Geometry check sheet. Reference: the model listing, model coordinates, mm. Face numbers are marked on the shaded views. A direction names the side the tool comes from. Coordinates: 2 decimals unless noted, no trailing zeros. Write each loop counter-clockwise with the first axis right and the second up, starting at its lowest first coordinate (ties: lowest second). Pieces come first, ordered by that corner, then holes. Notation, with made-up numbers: M 6,64.5 L 31,64.5 A24 cw 31,93.5 Z; hole C 30.5,0.25 d11. An arc over 180 degrees is marked long. Answer as a JSON object with one key per item and string values. Group by question number.
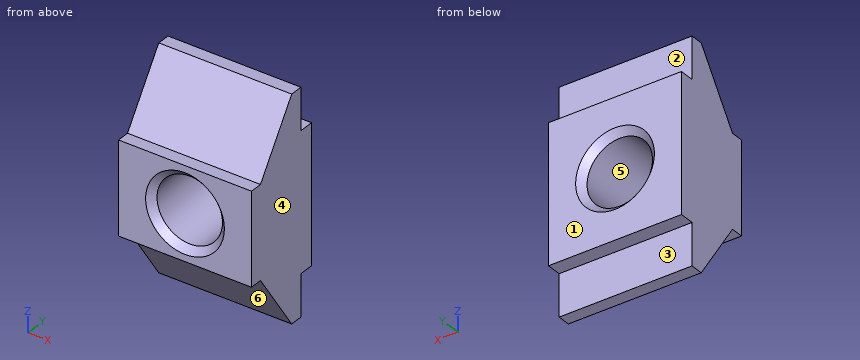
Autodesk Inventor part; units mm, degrees
ref_plane "TIN_4_XY" through (0, 8.5, 0) normal (0, 1, 0) x (1, 0, 0)
ref_plane "TIN_4_YZ" through (0, 8.5, 0) normal (1, 0, 0) x (0, 0, -1)
ref_plane "TIN_4_ZX" through (0, 8.5, 0) normal (0, 0, -1) x (0, 1, 0)
sketch "Skizze_1" plane through (0, 0, 0) normal (1, 0, 0) x (0, 1, 0)
  line L0 (5.7, 11.25) -> (1.275, 4.7)
  line L1 (1.275, 4.7) -> (0, 4.7)
  line L2 (0, 4.7) -> (0, -4.7)
  line L3 (0, -4.7) -> (1.275, -4.7)
  line L4 (1.275, -4.7) -> (5.7, -11.25)
  line L5 (5.7, -11.25) -> (7, -11.25)
  line L6 (7, -11.25) -> (7, -7)
  line L7 (7, -7) -> (8.5, -7)
  line L8 (8.5, -7) -> (8.5, 7)
  line L9 (8.5, 7) -> (7, 7)
  line L10 (7, 7) -> (7, 11.25)
  line L11 (7, 11.25) -> (5.7, 11.25)
extrude "Extrusion1" add sketch "Skizze_1" along normal mid plane 13.5
sketch "Skizze_2" plane through (0, 0, 0) normal (0, 0, 1) x (1, 0, 0)
  line L0 (0, 0) -> (0, 8.5)
  line L1 (0, 8.5) -> (4, 8.5)
  line L2 (4, 8.5) -> (3.3235, 7.8235)
  line L3 (3.3235, 7.8235) -> (3.3235, 0.6765)
  line L4 (3.3235, 0.6765) -> (4, 0)
  line L5 (4, 0) -> (0, 0)
  line L6 (0, 0) -> (0, 8.5)
revolve "Revolution1" cut sketch "Skizze_2" angle 360 about axis through (0, 0, 0) along (0, -1, 0)
thread "Thread1"
ref_plane "TIN_4_XY" through (0, 8.5, 0) normal (0, 1, 0) x (1, 0, 0)
ref_plane "TIN_4_YZ" through (0, 8.5, 0) normal (1, 0, 0) x (0, 0, -1)
ref_plane "TIN_4_ZX" through (0, 8.5, 0) normal (0, 0, -1) x (0, 1, 0)
properties part number "Robotunits TIN_4508"
1) Section check B-B (z = 0). Record the cut outline in (x, y).
2) Section check C-C (y = 6.75). Record the cut outline in (x, z), then the cut area to 3 significant figures.
3) Set-up check for the marked faces 1, 2 and 3: record each of +Z, -Z, +X, -X, +Y, -Y from which the full face is reachable in a straight line by a thin tool's end or side.
4) Section check D-D (x = -4.5). Record the cut outline in (y, z) (3 decimals), then the cut area to 3 significant figures.
5) Go/stop test with flat-tipped pins: pin 1 Ø1 at (x, y) = (0, 0.5) entering from -Z; pin 2 Ø2 at (x, y) = (-5, 1.5) entering from +Z; pin 3 Ø7.5 at (x, z) = (0, 0) entering from +Y. Record where each tip stops, or that it passes through.
6) Draft check along Z on the marked faces 4, 5 and 6. Enter one of: +Z half, -Z half, draft (parallel to the pull), parting line (faces both ways), or undercut.
7) Material ranges on probe 1 along Z at (x, y) = (0, 6); probe 2 along Z at (x, y) = (5.75, 7.5); probe 3 along Z at (x, y) = (0, 5.25), recorded low to high. Write a range as [from, to].
Entries:
{
 "1": {"outline": "M -6.75,0 L -4,0 L -3.32,0.68 L -3.32,7.82 L -4,8.5 L -6.75,8.5 Z; M 3.32,0.68 L 4,0 L 6.75,0 L 6.75,8.5 L 4,8.5 L 3.32,7.82 Z"},
 "2": {"outline": "M -6.75,-11.25 L 6.75,-11.25 L 6.75,11.25 L -6.75,11.25 Z; hole C 0,0 d6.65", "area": "269 mm^2"},
 "3": {"face 1": "+Z, -Z, +X, -X, +Y", "face 2": "+Z, +X, -X, +Y", "face 3": "-Z, +X, -X, +Y"},
 "4": {"outline": "M 0,-4.7 L 1.275,-4.7 L 5.7,-11.25 L 7,-11.25 L 7,-7 L 8.5,-7 L 8.5,7 L 7,7 L 7,11.25 L 5.7,11.25 L 1.275,4.7 L 0,4.7 Z", "area": "133 mm^2"},
 "5": {"pin 1": "z = -4.7", "pin 2": "z = 6.51", "pin 3": "y = 8.25"},
 "6": {"face 4": "draft", "face 5": "undercut", "face 6": "-Z half"},
 "7": {"probe 1": "[-11.25, -3.32], [3.32, 11.25]", "probe 2": "[-7, 7]", "probe 3": "[-10.58, -3.32], [3.32, 10.58]"}
}
